Solid Edge part; units mm, degrees
sketch "Sketch1" plane through (0, 0, 0) normal (0, 0, 1) x (1, 0, 0)
  circle A0 centre (99, 25.8394) radius 1.7
  line L0 (77, 19.8394) -> (105, 19.8394)
  line L1 (105, 19.8394) -> (105, 31.8394)
  line L2 (105, 31.8394) -> (77, 31.8394)
  line L3 (77, 31.8394) -> (77, 19.8394)
  circle A1 centre (83, 25.8394) radius 1.7
  dimension "D1" = 77
  dimension "D2" = 105
extrude "Protrusion1" add sketch "Sketch1" along normal blind 6
sketch "Sketch2" plane through (89, 25.8394, 6) normal (0, 0, 1) x (1, 0, 0)
  line L0 (7.15, 1.6454) -> (10, 3.2909)
  line L1 (10, 3.2909) -> (12.85, 1.6454)
  line L2 (12.85, 1.6454) -> (12.85, -1.6454)
  line L3 (12.85, -1.6454) -> (10, -3.2909)
  line L4 (10, -3.2909) -> (7.15, -1.6454)
  line L5 (7.15, -1.6454) -> (7.15, 1.6454)
  line L6 (-8.85, 1.6454) -> (-6, 3.2909)
  line L7 (-6, 3.2909) -> (-3.15, 1.6454)
  line L8 (-3.15, 1.6454) -> (-3.15, -1.6454)
  line L9 (-3.15, -1.6454) -> (-6, -3.2909)
  line L10 (-6, -3.2909) -> (-8.85, -1.6454)
  line L11 (-8.85, -1.6454) -> (-8.85, 1.6454)
extrude "ExtrudedCutout_1" cut sketch "Sketch2" against normal blind 3
properties material "ABS Plastic, high impact"
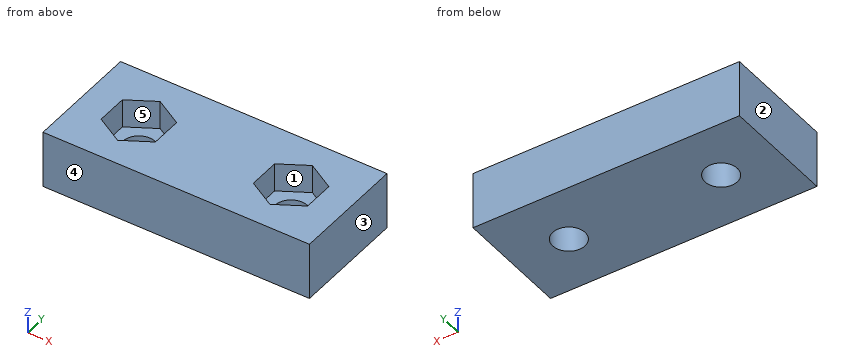
The listing builds one solid part. Answer for the finished solid, in the listing's coordinates (mm). Face numbers are marked on the shaded views. A direction names the side the tool comes from. Give positions to 0.01 mm unless a question says otherwise; leave off trailing zeros. Order: outer loops, then holes, each group sorted by start corner. A loop starts at its lowest first (then second) coordinate and runs counter-clockwise, first axis right, second up. Notation, with made-up numbers: (-33.5, 70) - (-0.5, 70) arc R20 cw to (-0.5, 89) - close; hole circle Ø6 at (75.5, 73). An arc over 180 degrees is marked (long way). Use one line per item in the form item = value. Start each with the question number.
(1) The mould has two halves that part along Y. Classify the marked faces 3, 4 and 5: released by +Y, released by -Y, zero draft, split by the parting line, or undercut.
(2) For the marked faces 1 and 2, determine the directions among +Z, -Z, +X, -X, +Y, -Y from which every point of the face is accessible in a straight line to the end or side of a thin tool.
(3) A flat-ended cylindrical pin translates along its axis: pin 1 Ø1.7 at (x, y) = (83, 24.5) entering from +Z. Find the tip coordinate at first contact, or state that the pin passes through.
(4) A cutting plane is placed at B-B, the plane x = 82.5. Write down the section's boundary in (y, z).
(5) A cutting plane is placed at A-A, the plane z = 3.85. Write down the section's boundary in (x, y).
(6) A cutting plane is placed at C-C, the plane y = 23.25. Write down the section's boundary in (x, z) (3 decimals), then the cut area to 3 significant figures.
(7) Consider line 1 (Y direction, x = 83, z = 1.15); line 2 (X direction, y = 23.25, z = 4.15) (3 decimals); line 3 (X direction, y = 25.25, z = 0.45). Determine where each line is inside the solid, lowest interval first. Write a range as from..to.
(8) A cutting plane is placed at D-D, the plane x = 98.25. Write down the section's boundary in (y, z).
Ans:
q1.face_3 = zero draft
q1.face_4 = released by -Y
q1.face_5 = undercut
q2.face_1 = +Z
q2.face_2 = +Z, -Z, -X, +Y, -Y
q3.pin_1 = 3
q4.outline = (19.84, 0) - (24.21, 0) - (24.21, 3) - (22.84, 3) - (22.84, 6) - (19.84, 6) - close; (27.46, 0) - (31.84, 0) - (31.84, 6) - (28.84, 6) - (28.84, 3) - (27.46, 3) - close
q5.outline = (77, 19.84) - (105, 19.84) - (105, 31.84) - (77, 31.84) - close; hole (80.15, 24.19) - (83, 22.55) - (85.85, 24.19) - (85.85, 27.48) - (83, 29.13) - (80.15, 27.48) - close; hole (96.15, 24.19) - (99, 22.55) - (101.85, 24.19) - (101.85, 27.48) - (99, 29.13) - (96.15, 27.48) - close
q6.outline = (77, 0) - (105, 0) - (105, 6) - (100.215, 6) - (100.215, 3) - (97.785, 3) - (97.785, 6) - (84.215, 6) - (84.215, 3) - (81.785, 3) - (81.785, 6) - (77, 6) - close
q6.area = 153 mm^2
q7.line_1 = 19.84..24.14, 27.54..31.84
q7.line_2 = 77..81.785, 84.215..97.785, 100.215..105
q7.line_3 = 77..81.41, 84.59..97.41, 100.59..105
q8.outline = (19.84, 0) - (24.31, 0) - (24.31, 3) - (22.98, 3) - (22.98, 6) - (19.84, 6) - close; (27.37, 0) - (31.84, 0) - (31.84, 6) - (28.7, 6) - (28.7, 3) - (27.37, 3) - close
